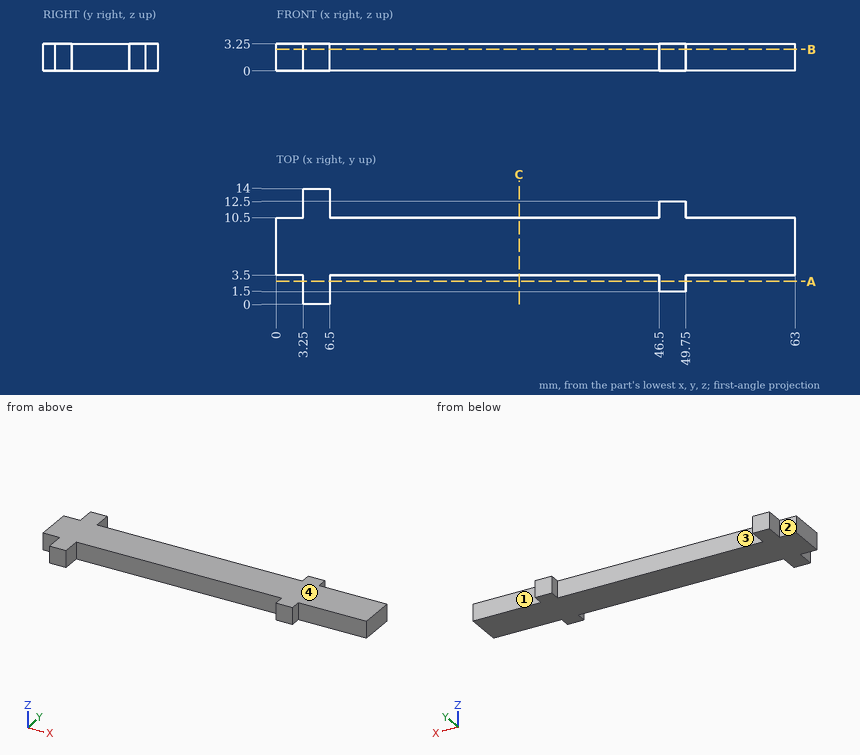
Can you work these out from the drawing? Everything is in mm from the part's minimum corner. A direction names the side the tool comes from. Round coordinates to 2 decimals unless told otherwise and drop trailing zeros. Loops run counter-clockwise (first coordinate to the right, second up) from the corner with the lowest first, then second, coordinate; pieces in that order, holes last. Notation, with made-up numbers: (-38.5, 69) - (-22.5, 69) arc R19 ccw to (-22.5, 74) - close; hole circle Ø3 at (70, 52.5). An arc over 180 degrees is marked (long way). Write item = value, one per line. Start each with the question number.
(1) If I drill on probe 1 along X at (y, z) = (11.5, 0.6); probe 2 along Y at (x, z) = (30, 2.9); probe 3 along Y at (x, z) = (47, 1.05), over which ranges is the centre line in solid material (lowest first)? Write a range as [from, to].
(2) If we section it at B-B (z = 2.6): Please give me the cut outline in (x, y).
(3) For the marked faces 1, 2, 3 and 4, which set-ups out of +Z, -Z, +X, -X, +Y, -Y let a thin tool reach every point of the face, with its end or its side?
(4) For P1, Ø1, axis at x = 27.5, z = 1, coming from the -Y side; P2, Ø1.6, axis at x = 56.5, z = 2.5, coming from the +Y side; P3, Ø1, axis at y = 11.5, z = 2, coming from the -X side, each with a flat end and sliding along its axis, tell me the tip position at first contact or that it passes through.
(5) If we section it at A-A (y = 2.75): Please give me the cut outline in (x, z).
(6) If we section it at C-C (x = 29.5): Please give me the cut outline in (y, z), and give its area (4 significant figures).
Ans:
q1.probe_1 = [3.25, 6.5], [46.5, 49.75]
q1.probe_2 = [3.5, 10.5]
q1.probe_3 = [1.5, 12.5]
q2.outline = (0, 3.5) - (3.25, 3.5) - (3.25, 0) - (6.5, 0) - (6.5, 3.5) - (46.5, 3.5) - (46.5, 1.5) - (49.75, 1.5) - (49.75, 3.5) - (63, 3.5) - (63, 10.5) - (49.75, 10.5) - (49.75, 12.5) - (46.5, 12.5) - (46.5, 10.5) - (6.5, 10.5) - (6.5, 14) - (3.25, 14) - (3.25, 10.5) - (0, 10.5) - close
q3.face_1 = +Z, -Z, +X, +Y
q3.face_2 = +Z, -Z, -X, +Y
q3.face_3 = +Z, -Z, +Y
q3.face_4 = +Z, +X, -X, +Y, -Y
q4.P1 = 3.5
q4.P2 = 10.5
q4.P3 = 3.25
q5.outline = (3.25, 0) - (6.5, 0) - (6.5, 3.25) - (3.25, 3.25) - close; (46.5, 0) - (49.75, 0) - (49.75, 3.25) - (46.5, 3.25) - close
q6.outline = (3.5, 0) - (10.5, 0) - (10.5, 3.25) - (3.5, 3.25) - close
q6.area = 22.75 mm²
